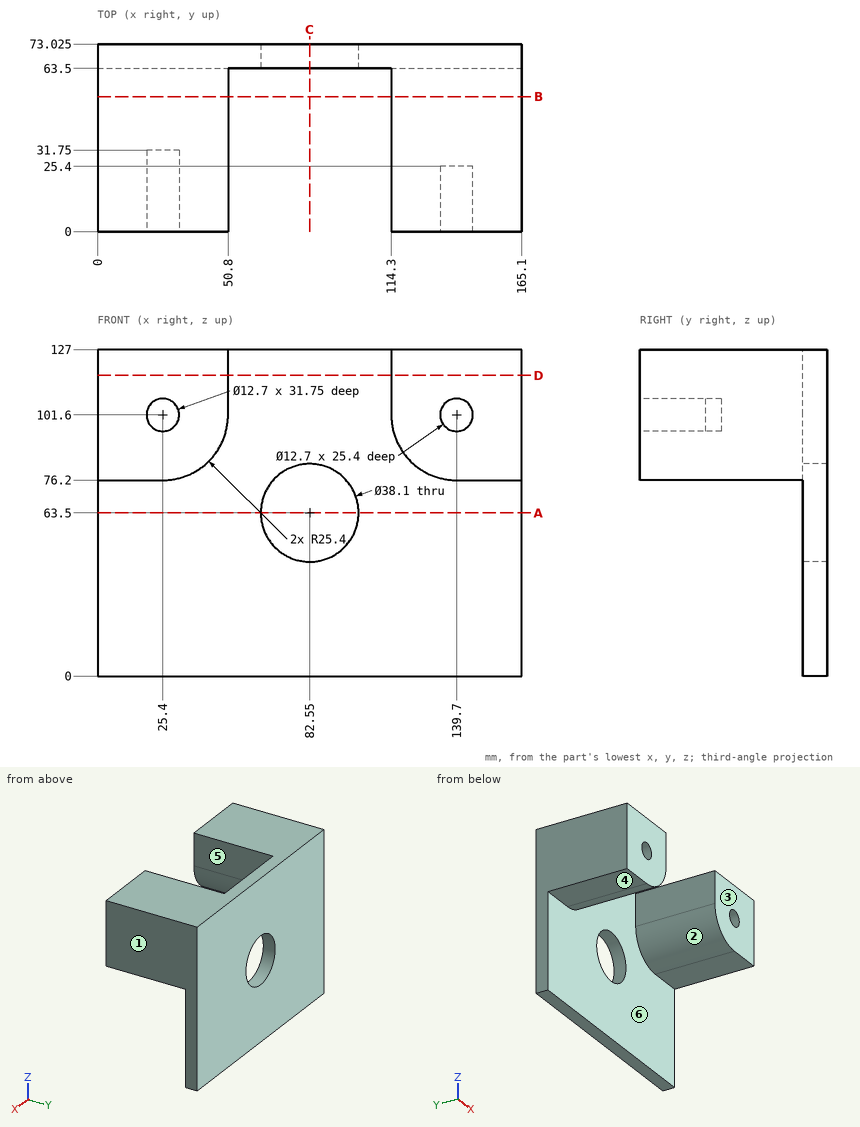
Check sheet for the drawn part. Datum: minimum x, y, z corner. Units: mm. A direction names the side the tool comes from. Coordinates: 2 decimals unless noted, no trailing zeros. Loops run counter-clockwise (first coordinate to the right, second up) from the corner with the lowest first, then second, coordinate; pieces in that order, holes last. Notation, with made-up numbers: (-26.5, 68.5) -> (-8.5, 68.5) arc R11 cw to (-8.5, 82.5) -> close; hole circle Ø9 at (-25, 56). An arc over 180 degrees is marked (long way). Answer as CSV lines item,"result".
1) Cross-section at D-D, the plane z = 117. Record the cut outline in (x, y) (3 decimals), then the cut area to 3 significant figures.
Found:
outline,"(0, 0) -> (50.8, 0) -> (50.8, 63.5) -> (114.3, 63.5) -> (114.3, 0) -> (165.1, 0) -> (165.1, 73.025) -> (0, 73.025) -> close"
area,"8,020 mm2"
2) Cross-section at C-C, the plane x = 82.55. Record the cut outline in (y, z) (3 decimals), then the cut area to 3 significant figures.
Found:
outline,"(63.5, 0) -> (73.025, 0) -> (73.025, 44.45) -> (63.5, 44.45) -> close; (63.5, 82.55) -> (73.025, 82.55) -> (73.025, 127) -> (63.5, 127) -> close"
area,"847 mm2"
3) Release check for a two-part mould opening along X. For the marked faces 1, 2 and 3 record: +X half, -X half, draft (parallel to the pull), parting line (faces both ways), or undercut.
Found:
face 1,"+X half"
face 2,"undercut"
face 3,"draft"
4) Depth check by flat-ended pin: pin 1 (5 mm diameter, centred on x = 94.5, z = 79.5, fed in from -Y); pin 2 (14 mm diameter, centred on x = 140.5, z = 99.5, fed in from -Y); pin 3 (20.5 mm diameter, centred on x = 147, y = 20, fed in from -Z); pin 4 (11.5 mm diameter, centred on x = 139.7, z = 101.6, fed in from -Y). Enter the tip coordinate at first touch or a pass-through.
Found:
pin 1,"stops at y = 63.5"
pin 2,"stops at y = 0"
pin 3,"stops at z = 76.2"
pin 4,"stops at y = 25.4"
5) Tool access check on the marked faces 4, 5 and 6. Record the directions out of +Z, -Z, +X, -X, +Y, -Y that give a thin tool (end or side, any length) a straight path to the whole face; none if there is none.
Found:
face 4,"-Z, +X, -X, -Y"
face 5,"+Z, -Z, -Y"
face 6,"-Z, -Y"
6) Thickness scan on L1, parallel to Z at x = 82, y = 67; L2, parallel to Z at x = 139.7, y = 15.5; L3, parallel to Y at x = 141, z = 64 (3 decimals). Record the ranges inside material, lowest first. Write a range as from..to.
Found:
L1,"z = 0..44.46, 82.54..127"
L2,"z = 76.2..95.25, 107.95..127"
L3,"y = 63.5..73.025"
7) Cross-section at B-B, the plane y = 52.5. Record the cut outline in (x, z).
Found:
outline,"(0, 76.2) -> (25.4, 76.2) arc R25.4 ccw to (50.8, 101.6) -> (50.8, 127) -> (0, 127) -> close; (114.3, 101.6) arc R25.4 ccw to (139.7, 76.2) -> (165.1, 76.2) -> (165.1, 127) -> (114.3, 127) -> close"
8) Cross-section at A-A, the plane z = 63.5. Record the cut outline in (x, y) (3 decimals).
Found:
outline,"(0, 63.5) -> (63.5, 63.5) -> (63.5, 73.025) -> (0, 73.025) -> close; (101.6, 63.5) -> (165.1, 63.5) -> (165.1, 73.025) -> (101.6, 73.025) -> close"
